Source: CAD feature listing. Evaluate the final solid. Frame: model axes, mm. Face numbers are marked on the shaded views. Give positions to 0.01 mm unless a question says otherwise; leave off trailing zeros. Write each loop counter-clockwise with the first axis right and the second up, starting at its lowest first coordinate (ties: lowest second). Pieces come first, ordered by that corner, then holes. Notation, with made-up numbers: M -13.75,31.25 L -0.75,31.25 A31 ccw -0.75,56.25 Z; hole C 6,-9.75 d10. An arc over 180 degrees is marked long. Return JSON: item names as keys, results as strings.
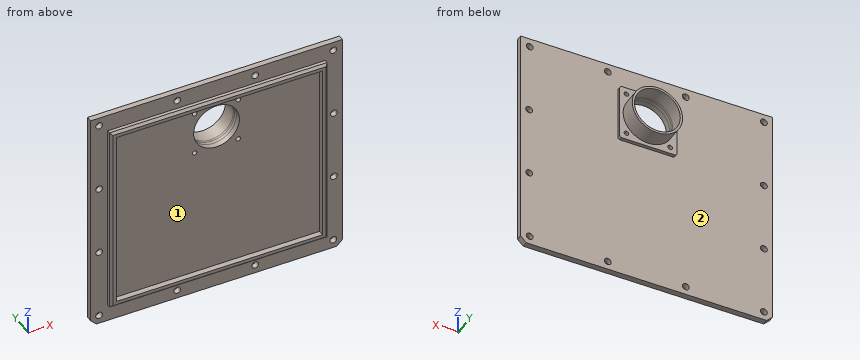
```python
from build123d import *
from build123d.topology import SkipClean

# Parameters (mm, degrees)
SKETCH1_R           = 3
SKETCH1_R_2         = 20
BOSS_EXTRUDE1_DEPTH = 5
CHAMFER1_SIZE       = 5
BOSS_EXTRUDE3_DEPTH = 3
SKETCH3_R           = 22
SKETCH3_R_2         = 20
BOSS_EXTRUDE4_DEPTH = 15
FILLET2_R           = 2
BOSS_EXTRUDE5_DEPTH = 5
SKETCH6_R           = 20
CUT_EXTRUDE1_DEPTH  = 5
SKETCH7_R           = 2
CUT_EXTRUDE2_DEPTH  = 10
CHAMFER2_SIZE       = 2


with BuildPart() as part:
    # Sketch1 → Boss-Extrude1 (new body)
    with BuildSketch(Plane(origin=(0, 0, 0), x_dir=(1, 0, 0), z_dir=(0, 1, 0))):
        Polygon((110, -150), (110, 50), (0, 50), (-110, 50), (-110, -150), align=None)
        with Locations(Location((-102.5, 42.5, 0), (0, 0, 270))):
            Circle(SKETCH1_R, mode=Mode.SUBTRACT)
        with Locations(Location((-34.33, 42.5, 0), (0, 0, 270))):
            Circle(SKETCH1_R, mode=Mode.SUBTRACT)
        with Locations(Location((33.84, 42.5, 0), (0, 0, 270))):
            Circle(SKETCH1_R, mode=Mode.SUBTRACT)
        with Locations(Location((102.01, 42.5, 0), (0, 0, 270))):
            Circle(SKETCH1_R, mode=Mode.SUBTRACT)
        with Locations(Location((-34.33, -142.5, 0), (0, 0, 270))):
            Circle(SKETCH1_R, mode=Mode.SUBTRACT)
        with Locations(Location((33.84, -142.5, 0), (0, 0, 270))):
            Circle(SKETCH1_R, mode=Mode.SUBTRACT)
        with Locations(Location((102.01, -142.5, 0), (0, 0, 270))):
            Circle(SKETCH1_R, mode=Mode.SUBTRACT)
        with Locations(Location((-102.5, -142.5, 0), (0, 0, 270))):
            Circle(SKETCH1_R, mode=Mode.SUBTRACT)
        with Locations(Location((-102.5, -19.17, 0), (0, 0, 270))):
            Circle(SKETCH1_R, mode=Mode.SUBTRACT)
        with Locations(Location((-102.5, -80.84, 0), (0, 0, 270))):
            Circle(SKETCH1_R, mode=Mode.SUBTRACT)
        with Locations(Location((102.5, -19.17, 0), (0, 0, 270))):
            Circle(SKETCH1_R, mode=Mode.SUBTRACT)
        with Locations(Location((102.5, -80.84, 0), (0, 0, 270))):
            Circle(SKETCH1_R, mode=Mode.SUBTRACT)
        with Locations(Location((0, -105, 0), (0, 0, 270))):
            Circle(SKETCH1_R_2, mode=Mode.SUBTRACT)
    extrude(amount=BOSS_EXTRUDE1_DEPTH)

    # Chamfer1
    chamfer1_edges = [part.edges().sort_by_distance(p)[0] for p in [
        (110, 2.5, -50),
        (-110, 2.5, -50),
    ]]
    chamfer(chamfer1_edges, length=CHAMFER1_SIZE)

    # Sketch2 → Boss-Extrude3 (add)
    with BuildSketch(Plane(origin=(0, 5, 0), x_dir=(1, 0, 0), z_dir=(0, 1, 0))):
        Polygon((0, -130), (-25, -130), (-25, -80), (25, -80), (25, -130), align=None)
    extrude(amount=BOSS_EXTRUDE3_DEPTH)

    # Sketch3 → Boss-Extrude4 (add)
    with BuildSketch(Plane(origin=(0, 8, 0), x_dir=(1, 0, 0), z_dir=(0, 1, 0))):
        with Locations(Location((0, -105, 0), (0, 0, 90))):
            Circle(SKETCH3_R)
        with Locations(Location((0, -105, 0), (0, 0, 90))):
            Circle(SKETCH3_R_2, mode=Mode.SUBTRACT)
    extrude(amount=BOSS_EXTRUDE4_DEPTH)

    # Fillet2
    fillet2_edges = [part.edges().sort_by_distance(p)[0] for p in [
        (-25, 6.5, 80),
        (-25, 6.5, 130),
        (25, 6.5, 130),
        (25, 6.5, 80),
    ]]
    fillet(fillet2_edges, radius=FILLET2_R)

    # Sketch4 → Boss-Extrude5 (add)
    with BuildSketch(Plane.XZ):
        Polygon((95, 135), (0, 135), (-95, 135), (-95, -35), (95, -35), align=None)
        Polygon((-90, 130), (0, 130), (90, 130), (90, -30), (-90, -30), align=None, mode=Mode.SUBTRACT)
    extrude(amount=BOSS_EXTRUDE5_DEPTH)

    # Sketch6 → Cut-Extrude1 (cut)
    with SkipClean():  # the faces are left unmerged after this step: merging them gives an invalid solid
        with BuildSketch(Plane.XZ.offset(-5)):
            with Locations(Location((0, 105, 0), (0, 0, 90))):
                Circle(SKETCH6_R)
        extrude(amount=-CUT_EXTRUDE1_DEPTH, mode=Mode.SUBTRACT)

    # Sketch7 → Cut-Extrude2 (cut)
    with BuildSketch(Plane(origin=(0, 8, 0), x_dir=(1, 0, 0), z_dir=(0, 1, 0))):
        with Locations(Location((19.091883092, -124.091883092, 0), (0, 0, 270))):
            Circle(SKETCH7_R)
        with Locations(Location((-19.091883092, -124.091883092, 0), (0, 0, 270))):
            Circle(SKETCH7_R)
        with Locations(Location((-19.091883092, -85.908116908, 0), (0, 0, 270))):
            Circle(SKETCH7_R)
        with Locations(Location((19.091883092, -85.908116908, 0), (0, 0, 270))):
            Circle(SKETCH7_R)
    extrude(amount=-CUT_EXTRUDE2_DEPTH, mode=Mode.SUBTRACT)

    # Chamfer2
    chamfer2_edges = [part.edges().sort_by_distance(p)[0] for p in [
        (0, -5, 135),
        (-95, -5, 50),
        (0, -5, -35),
        (95, -5, 50),
    ]]
    chamfer(chamfer2_edges, length=CHAMFER2_SIZE)


solid = part.part
```
1) Cut plane B-B, the plane z = 105. Return the cut outline in (x, y), then the cut area to 3 significant figures.
Numbers:
{"outline": "M -110,0 L -95,0 L -95,-3 L -93,-5 L -90,-5 L -90,0 L -20,0 L -20,23 L -22,23 L -22,8 L -25,8 L -25,5 L -110,5 Z; M 20,0 L 90,0 L 90,-5 L 93,-5 L 95,-3 L 95,0 L 110,0 L 110,5 L 25,5 L 25,8 L 22,8 L 22,23 L 20,23 Z", "area": "1,040 mm²"}
2) Draft query along X for the marked faces 1 and 2. Return one class per face: released by +X, released by -X, zero draft, split by the parting line, or undercut.
Numbers:
{"face 1": "undercut", "face 2": "zero draft"}
3) Cut plane A-A, the plane x = 33.84. Return the cut outline in (y, z), then the cut area to 3 significant figures.
Numbers:
{"outline": "M -5,-33 L -3,-35 L 0,-35 L 0,-39.5 L 5,-39.5 L 5,139.5 L 0,139.5 L 0,135 L -3,135 L -5,133 L -5,130 L 0,130 L 0,-30 L -5,-30 Z; M 0,-50 L 5,-50 L 5,-45.5 L 0,-45.5 Z; M 0,145.5 L 5,145.5 L 5,150 L 0,150 Z", "area": "986 mm²"}
4) Cut plane C-C, the plane x = -102.5. Return the cut outline in (y, z).
Numbers:
{"outline": "M 0,-50 L 5,-50 L 5,-45.5 L 0,-45.5 Z; M 0,-39.5 L 5,-39.5 L 5,16.17 L 0,16.17 Z; M 0,22.17 L 5,22.17 L 5,77.84 L 0,77.84 Z; M 0,83.84 L 5,83.84 L 5,139.5 L 0,139.5 Z; M 0,145.5 L 5,145.5 L 5,150 L 0,150 Z"}
5) Line query: line 1 (X direction, y = 4.05, z = 19.17); line 2 (X direction, y = 3.5, z = -42.5); line 3 (X direction, y = 18.5, z = 105). Output: solid intervals per line, ascending. Write a range as [from, to].
Numbers:
{"line 1": "x = [-110, -105.5], [-99.5, 99.5], [105.5, 110]", "line 2": "x = [-110, -105.5], [-99.5, -37.33], [-31.33, 30.84], [36.84, 99.01], [105.01, 110]", "line 3": "x = [-22, -20], [20, 22]"}
6) Cut plane D-D, the plane z = -25.5. Return the cut outline in (x, y), then the cut area to 3 significant figures.
Numbers:
{"outline": "M -110,0 L -95,0 L -95,-3 L -93,-5 L -90,-5 L -90,0 L 90,0 L 90,-5 L 93,-5 L 95,-3 L 95,0 L 110,0 L 110,5 L -110,5 Z", "area": "1,150 mm²"}
7) Contact query for flat-ended pins moving along their axis: pin 1 Ø9.5 at (x, z) = (33.84, -42.5) entering from +Y; pin 2 Ø3.5 at (x, z) = (102.5, 80.84) entering from +Y; pin 3 Ø1 at (y, z) = (14, 112.5) entering from -X; pin 4 Ø8 at (x, z) = (-102.5, -42.5) entering from -Y. Output: stop coordinate, or through.
Numbers:
{"pin 1": "stops at y = 5", "pin 2": "passes through", "pin 3": "stops at x = -20.86", "pin 4": "stops at y = 0"}
